```python
from build123d import *

# Parameters (mm, degrees)
SCHIZZO1_W                   = 50
SCHIZZO1_H                   = 80
ESTRUSIONE_ESTRUSIONE1_DEPTH = 3
SCHIZZO2_W                   = 3
SCHIZZO2_H                   = 2.857142857
ESTRUSIONE_ESTRUSIONE2_DEPTH = 3
SCHIZZO3_W                   = 3
SCHIZZO3_H                   = 5.714285715
ESTRUSIONE_ESTRUSIONE3_DEPTH = 3
RIPETIZIONE_A_L1_COUNT       = 6
RIPETIZIONE_A_L1_PITCH       = 11.428571
SCHIZZO4_W                   = 6.25
SCHIZZO4_H                   = 3
ESTRUSIONE_ESTRUSIONE4_DEPTH = 3
RIPETIZIONE_A_L2_COUNT       = 4
RIPETIZIONE_A_L2_PITCH       = 12.5


with BuildPart() as part:
    # Schizzo1 → Estrusione-Estrusione1 (new body)
    with BuildSketch(Plane(origin=(0, 0, 0), x_dir=(0, 0, -1), z_dir=(1, 0, 0))):
        with Locations((25, 40)):
            Rectangle(SCHIZZO1_W, SCHIZZO1_H)
    extrude(amount=ESTRUSIONE_ESTRUSIONE1_DEPTH)

    # Schizzo2 → Estrusione-Estrusione2 (add)
    with BuildSketch(Plane(origin=(3, 0, 0), x_dir=(0, 0, -1), z_dir=(1, 0, 0))):
        with Locations((-1.5, 78.571428572)):
            Rectangle(SCHIZZO2_W, SCHIZZO2_H)
        with Locations((51.5, 78.571428572)):
            Rectangle(SCHIZZO2_W, SCHIZZO2_H)
        with Locations((51.5, 1.428571429)):
            Rectangle(SCHIZZO2_W, SCHIZZO2_H)
        with Locations((-1.5, 1.428571429)):
            Rectangle(SCHIZZO2_W, SCHIZZO2_H)
    extrude(amount=-ESTRUSIONE_ESTRUSIONE2_DEPTH)

    # Schizzo3 → Estrusione-Estrusione3 (add)
    with BuildSketch(Plane(origin=(3, 0, 0), x_dir=(0, 0, -1), z_dir=(1, 0, 0))):
        with Locations((-1.5, 68.571428572)):
            Rectangle(SCHIZZO3_W, SCHIZZO3_H)
        with Locations((51.5, 68.571428572)):
            Rectangle(SCHIZZO3_W, SCHIZZO3_H)
    estrusione_estrusione3 = extrude(amount=-ESTRUSIONE_ESTRUSIONE3_DEPTH)

    # Ripetizione a L1: Estrusione-Estrusione3 ×6
    with Locations(*[(0, -i * RIPETIZIONE_A_L1_PITCH, 0) for i in range(1, RIPETIZIONE_A_L1_COUNT)]):
        add(estrusione_estrusione3)

    # Schizzo4 → Estrusione-Estrusione4 (add)
    with BuildSketch(Plane(origin=(3, 0, 0), x_dir=(0, 0, -1), z_dir=(1, 0, 0))):
        with Locations((6.25, 81.5)):
            Rectangle(SCHIZZO4_W, SCHIZZO4_H)
        with Locations((6.25, -1.5)):
            Rectangle(SCHIZZO4_W, SCHIZZO4_H)
    estrusione_estrusione4 = extrude(amount=-ESTRUSIONE_ESTRUSIONE4_DEPTH)

    # Ripetizione a L2: Estrusione-Estrusione4 ×4
    with Locations(*[(0, 0, -i * RIPETIZIONE_A_L2_PITCH) for i in range(1, RIPETIZIONE_A_L2_COUNT)]):
        add(estrusione_estrusione4)


solid = part.part
```
The listing builds one solid part. Answer for the finished solid, in the listing's coordinates (mm). A direction names the side the tool comes from. Give positions to 0.01 mm unless a question says otherwise; leave off trailing zeros. Order: outer loops, then holes, each group sorted by start corner. A loop starts at its lowest first (then second) coordinate and runs counter-clockwise, first axis right, second up. Notation, with made-up numbers: (-0.5, 13) - (14.5, 13) arc R11 cw to (14.5, 32) - close; hole circle Ø6 at (76.25, -23.75). An arc over 180 degrees is marked (long way). Answer in a Markdown table with one row per item. Add a question column.
Q1. The part is cut by section A-A (z = -24.5). Determine the outline of the cut face in (x, y).
Q2. Find the intervals of material crossed by line 1 along Z through (x, y) = (2.05, 19); line 2 along Y through (x, z) = (2.8, -2.5), in increasing order. Write a range as [from, to].
Q3. For a pull along Y with two mould halves and no side action, classify faces 5 (the flat face through (2, 79, 3)), 6 (the flat face through (2, -3, -31)), 7 (the flat face through (2, 54.286, 2)), 8 (the flat face through (1, 6, -50)) as released by +Y, released by -Y, zero draft, split by the parting line, or undercut.
Q4. Given P1, Ø1.5, axis at x = 2, z = -24.5, coming from the +Y side; P2, Ø0.9, axis at x = 1.5, y = 50, coming from the -Z side; P3, Ø0.9, axis at x = 2, y = 82, coming from the +Z side (3 decimals), each flat-ended and moving along its own axis, determine where each tip first touches the part or whether it passes through.
Q5. Which of the six approach directions +Z, -Z, +X, -X, +Y, -Y give full straight-line access (tool end or side, diameter ignored) to faces 1 (the flat face through (2, -2, -40.625)), 2 (the flat face through (1, 40, -50)), 3 (the flat face through (2, -2, -3.125)), 4 (the flat face through (1, 40, 0))?
Determined:
| question | item | result |
|---|---|---|
| 1 | outline | (0, 0) - (3, 0) - (3, 80) - (0, 80) - close |
| 2 | line 1 | z = [-50, 0] |
| 2 | line 2 | y = [0, 80] |
| 3 | face 5 | zero draft |
| 3 | face 6 | released by -Y |
| 3 | face 7 | undercut |
| 3 | face 8 | undercut |
| 4 | P1 | stops at y = 80 |
| 4 | P2 | stops at z = -50 |
| 4 | P3 | stops at z = -3.125 |
| 5 | face 1 | +X, -X, -Y |
| 5 | face 2 | -Z, +X, -X |
| 5 | face 3 | +Z, +X, -X, -Y |
| 5 | face 4 | +Z, +X, -X |
